Here's how the part is built. I have some questions about the finished solid (model axes, mm). Face numbers are marked on the shaded views. A direction names the side the tool comes from. Round coordinates to 2 decimals unless told otherwise and drop trailing zeros. Write each loop counter-clockwise with the first axis right and the second up, starting at its lowest first coordinate (ties: lowest second). Pieces come first, ordered by that corner, then holes. Notation, with made-up numbers: M 64.5,81 L 89.5,81 A14 cw 89.5,102 Z; hole C 21,39 d7. An arc over 180 degrees is marked long. Use a Markdown table: item, result. Add a question column.
```python
from build123d import *

# Parameters (mm, degrees)
F1_DEPTH = 8
F2_SIZE  = 1


with BuildPart() as f1:
    # F0 (on Right) → F1 (new body)
    with BuildSketch(Plane.YZ):
        Polygon((-17.413627, 2.447326), (0, 0), (0, -7), (8, -7), (8, 9.5), (-1.095375, 10.778272), (-2, 4.341529), (-11.902681, 5.73326), (-10.998056, 12.170003), (-15.949396, 12.865868), align=None)
    extrude(amount=F1_DEPTH)

    # F2
    f2_edges = [f1.edges().sort_by_distance(p)[0] for p in [
        (4, 8, -7),
    ]]
    chamfer(f2_edges, length=F2_SIZE)


solid = f1.part
```
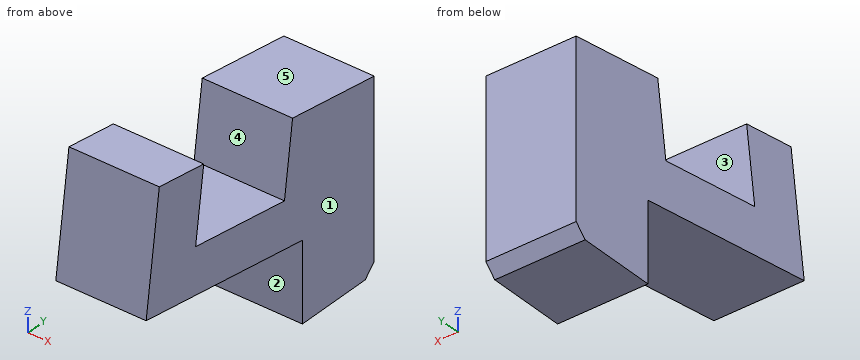
Item 1: For pin 1 Ø3.5 at (x, z) = (4.5, -4) entering from -Y; pin 2 Ø3 at (x, z) = (3.5, 7.5) entering from -Y; pin 3 Ø1.5 at (x, y) = (2.5, -3) entering from -Z; pin 4 Ø1 at (y, z) = (-11, 8) entering from +X, each with a flat end and sliding along its axis, tell me the tip position at first contact or that it passes through.
Item 2: Imagine slicing it at D-D on y = 2. List the corners of the cut face in (x, z) for me.
Item 3: Imagine slicing it at C-C on z = -4.5. List the corners of the cut face in (x, y) for me, plus the area to 3 significant figures.
Item 4: Imagine slicing it at A-A on z = 10.5. List the corners of the cut face in (x, y) for me.
Item 5: Imagine slicing it at B-B on x = 4. List the corners of the cut face in (y, z) for me, plus the area to 3 significant figures.
Item 6: I need wall thicknesses on probe 1 along Y at (x, z) = (2.75, 7.75); probe 2 along Y at (x, z) = (4.5, -1.25); probe 3 along Z at (x, y) = (1, -12.75). Which ranges of each line are inside material? Lowest first, please. Write a range as from..to.
Item 7: On a 3-axis mill with a long thin cutter (end or side, diameter ignored), from which of +Z, -Z, +X, -X, +Y, -Y can I reach the whole of each face in a straight line? I mean the marked faces 1, 2, 3, 4 and 5. Say none if no direction works.
The answers:
| question | item | result |
|---|---|---|
| 1 | pin 1 | y = 0 |
| 1 | pin 2 | y = -16.91 |
| 1 | pin 3 | z = 0.32 |
| 1 | pin 4 | through |
| 2 | outline | M 0,-7 L 8,-7 L 8,10.34 L 0,10.34 Z |
| 3 | outline | M 0,0 L 8,0 L 8,8 L 0,8 Z |
| 3 | area | 64.0 mm² |
| 4 | outline | M 0,-16.28 L 8,-16.28 L 8,-11.23 L 0,-11.23 Z; M 0,-1.13 L 8,-1.13 L 8,0.88 L 0,0.88 Z |
| 5 | outline | M -17.41,2.45 L 0,0 L 0,-7 L 7,-7 L 8,-6 L 8,9.5 L -1.1,10.78 L -2,4.34 L -11.9,5.73 L -11,12.17 L -15.95,12.87 Z |
| 5 | area | 248 mm² |
| 6 | probe 1 | -16.67..-11.62, -1.52..8 |
| 6 | probe 2 | 0..8 |
| 6 | probe 3 | 1.79..12.42 |
| 7 | face 1 | +Z, -Z, +X, +Y, -Y |
| 7 | face 2 | -Z, +X, -X, -Y |
| 7 | face 3 | +X, -X |
| 7 | face 4 | +Z, +X, -X |
| 7 | face 5 | +Z, +X, -X, +Y |
